Source: CAD feature listing. Evaluate the final solid. Frame: model axes, mm. Face numbers are marked on the shaded views. A direction names the side the tool comes from. Coordinates: 2 decimals unless noted, no trailing zeros. Write each loop counter-clockwise with the first axis right and the second up, starting at its lowest first coordinate (ties: lowest second). Pieces come first, ordered by that corner, then holes. Notation, with made-up numbers: (19.25, -17.75) - (41.25, -17.75) arc R15 cw to (41.25, -11.75) - close; hole circle Ø2 at (18, 65). An arc over 180 degrees is marked (long way). One line per item, written item: value.
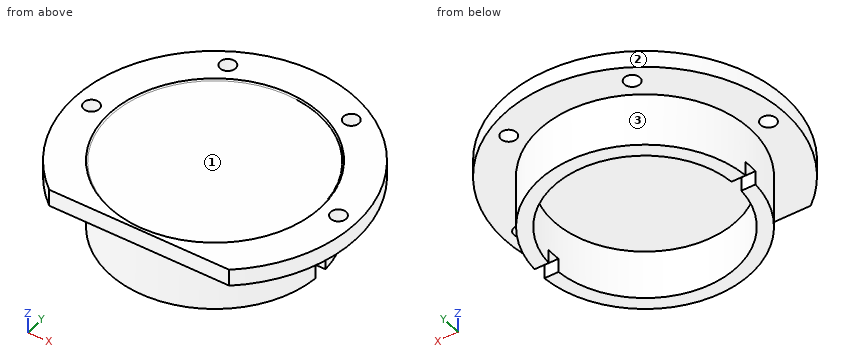
Autodesk Inventor part; units mm, degrees
ref_plane "工作平面1" through (0, 0, 0) normal (0, 0, 1) x (1, 0, 0)
ref_plane "YZ Plane" through (0, 0, 0) normal (1, 0, 0) x (0, 1, 0)
ref_plane "XZ Plane" through (0, 0, 0) normal (0, 1, 0) x (-1, 0, 0)
ref_plane "工作平面1" through (0, 0, 0) normal (0, 0, 1) x (1, 0, 0)
sketch "草图1" plane through (0, 0, 0) normal (0, 0, 1) x (1, 0, 0)
  arc A0 (9.993, -85.0026) -> (-35, 93.8712) centre (-50, -4.9974) ccw construction
  arc A1 (-50, -79.9974) -> (-50, 70.0026) centre (-50, -4.9974) ccw construction
  line L0 (-50, -79.9974) -> (-50, -85.0026) construction
  line L1 (-35, -85.0026) -> (-50, -85.0026) construction
  line L2 (-35, -95.0026) -> (-35, -85.0026) construction
  line L3 (9.993, -95.0026) -> (-35, -95.0026) construction
  line L4 (9.993, -95.0026) -> (9.993, -85.0026) construction
  arc A2 (9.993, -85.0026) -> (-35, 93.8712) centre (-50, -4.9974) ccw construction
  line L5 (-35, 93.8712) -> (-35, 95.0026) construction
  line L6 (-35, 95.0026) -> (-50, 95.0026) construction
  line L7 (-50, 95.0026) -> (-50, 70.0026) construction
  arc A3 (13.8044, -81.9974) -> (-113.8044, -81.9974) centre (-50, -4.9974) ccw
  line L8 (-113.8044, -81.9974) -> (13.8044, -81.9974)
  circle A4 centre (-50, -4.9974) radius 87.5 construction
  line L9 (-162.5015, -4.9974) -> (70.6652, -4.9974) construction
  circle A5 centre (-137.5, -4.9974) radius 5.5
  circle A6 centre (-93.75, -80.7746) radius 5.5 construction
  circle A7 centre (-6.25, -80.7746) radius 5.5 construction
  circle A8 centre (37.5, -4.9974) radius 5.5
  circle A9 centre (-6.25, 70.7799) radius 5.5
  circle A10 centre (-93.75, 70.7799) radius 5.5
  point P0 (0, 0)
  point P1 (-50, -81.9974)
  dimension "d1" = 175
  dimension "d0" = 2
  dimension "d2" = 11
  dimension "d5" = 360
extrude "拉伸1" add sketch "草图1" along normal blind 12
sketch "草图2" plane through (0, 0, 0) normal (0, 0, -1) x (-1, 0, 0)
  arc A0 (113.8044, -81.9974) -> (-13.8044, -81.9974) centre (50, -4.9974) ccw construction
  circle A1 centre (50, -4.9974) radius 75
  circle A2 centre (50, -4.9974) radius 65
  point P0 (0, 0)
  dimension "d9" = 150
  dimension "d10" = 10
extrude "拉伸2" add sketch "草图2" along normal blind 38
sketch "草图3" plane through (0, 0, 12) normal (0, 0, 1) x (1, 0, 0)
  arc A0 (13.8044, -81.9974) -> (-113.8044, -81.9974) centre (-50, -4.9974) ccw construction
  circle A1 centre (-50, -4.9974) radius 75
  circle A2 centre (-137.5, -4.9974) radius 5.5 construction
  point P0 (0, 0)
  dimension "d13" = 150
extrude "拉伸3" cut sketch "草图3" against normal blind 1
fillet "圆角1" radius 1 1 edges at (-125, -4.9974, 11)
sketch "草图4" plane through (-50, -4.9974, -38) normal (0, 0, -1) x (-1, 0, 0)
  line L0 (100, 5) -> (-100, 5)
  line L1 (-100, 5) -> (-100, -5)
  line L2 (-100, -5) -> (100, -5)
  line L3 (100, -5) -> (100, 5)
  circle A0 centre (0, 0) radius 65 construction
  point P0 (-50, 4.9974)
  point P1 (100, 0)
  point P2 (0, -5)
  dimension "d17" = 10
  dimension "d18" = 200
extrude "拉伸4" cut sketch "草图4" against normal blind 10
sketch "草图5" plane through (-50, -4.9974, 0) normal (0, 0, -1) x (-1, 0, 0)
  circle A0 centre (0, 0) radius 65
  point P0 (-50, 4.9974)
extrude "拉伸5" add sketch "草图5" along normal blind 3
properties part number "轴承端盖3"
1) Section query A-A on x = -137.5. Output: boundary loops of the cut face in (y, z).
Values found:
outline: (-53.41, 0) - (-10.5, 0) - (-10.5, 12) - (-53.41, 12) - close; (0.5, 0) - (43.41, 0) - (43.41, 12) - (0.5, 12) - close
2) Contact query for flat-ended pins moving along their axis: P1, Ø10, axis at y = 69.5, z = -30, coming from the +X side; P2, Ø4, axis at x = -18, z = -21, coming from the -Y side; P3, Ø3, axis at x = 22.5, y = -3.5, coming from the -Z side. Output: stop coordinate, or through.
Values found:
P1: x = -21.8
P2: y = -73.74
P3: z = -28
3) Section query C-C on z = -18. Output: boundary loops of the cut face in (x, y).
Values found:
outline: circle Ø150 at (-50, -5); hole circle Ø130 at (-50, -5)
4) Reachability of the marked faces 1, 2 and 3 from +Z, -Z, +X, -X, +Y, -Y: full face, straight path, thin tool, end or side. Return the list, or none.
Values found:
face 1: +Z
face 2: +Z, -Z
face 3: -Z
5) Material intervals for line 1 (Z direction, x = -48, y = -2); line 2 (Z direction, x = -121.5, y = -53.5); line 3 (Y direction, x = -76, z = -8), sorted ascending.
Values found:
line 1: -3 to 11
line 2: 0 to 12
line 3: -75.35 to -64.57, 54.58 to 65.35
